Design review of the part built by this model. Coordinates are the model's own, in mm. A direction names the side the tool comes from. Coordinates: 2 decimals unless noted, no trailing zeros. Write each loop counter-clockwise with the first axis right and the second up, starting at its lowest first coordinate (ties: lowest second). Pieces come first, ordered by that corner, then holes.
Q1. Take a section at D-D, the plane z = -8. Write out the cut boundary in (x, y).
Q2. The part is to be moulded in two halves that separate along Y. For faces 1 (the flat face through (-20, 14, -25)), 2 (the flat face through (-0.706, -46.367, 5.514)), 3 (the flat face through (-5, 27.3, -11)), say which applies: released by +Y, released by -Y, zero draft, split by the parting line, or undercut.
Q3. For pin 1 Ø0.6 at (x, z) = (-21, -27.5) entering from -Y; pin 2 Ø21 at (x, y) = (7.5, -3.5) entering from +Z; pin 3 Ø0.9 at (y, z) = (14.5, -25.5) entering from +X, all flat-tipped, find the tip position at first contact; note any pin that passes through.
Q4. Take a section at C-C, the plane x = 2.5. Write out the cut boundary in (y, z).
Q5. Take a section at A-A, the plane x = -15. Write out the cut boundary in (y, z).
Q6. For L1, parallel to Z at x = -9, y = 11.5; L2, parallel to Y at x = 6.5, z = 4; L3, parallel to Z at x = 7.5, y = 14.5, list the stretches that pass through material, from the lowest coordinate up.
Q7. For faces 4 (the flat face through (-21.014, 17.528, -12.159)), 5 (the flat face through (-11, 14, -20.21)), 6 (the flat face through (-21, 12.15, -25)), 7 (the flat face through (7, -20.2, 11)), 8 (the flat face through (-20, -8, -28)), list the 3-axis set-ups (+Z, -Z, +X, -X, +Y, -Y) from which the entire face can be reached by the end or side of a thin tool; tool diameter is ignored.
Q8. Take a section at B-B, the plane y = 16.5. Write out the cut boundary in (x, z).
from build123d import *

# Parameters (mm, degrees)
F1_DEPTH  = 20
F0_W      = 12
F0_H      = 10
F2_DEPTH  = 20
F4_DEPTH  = 2
F8_DEPTH  = 3
F10_DEPTH = 2


with BuildPart() as f1:
    # F0 (on Right) → F1 (new body)
    with BuildSketch(Plane.YZ):
        with BuildLine():
            ThreePointArc((-9.7216395426, -22.7567306352), (3.9984194059, -3.7830302321), (27.3, -6.0803474404))
            Line((27.3, -6.0803474404), (27.3, 1.2904210016))
            Line((27.3, 1.2904210016), (20.2, 1.2904210016))
            Line((20.2, 1.2904210016), (-20.2, 1.2904210016))
            Line((-20.2, 1.2904210016), (-27.3, 1.2904210016))
            Line((-27.3, 1.2904210016), (-33.1852941176, 1.2904210016))
            Line((-33.1852941176, 1.2904210016), (-14.8038696072, -17.5481150452))
            Line((-14.8038696072, -17.5481150452), (-9.7216395426, -22.7567306352))
        make_face()
        with BuildLine():
            Line((-42.245950674, 1.2904210016), (-33.1852941176, 1.2904210016))
            Line((-33.1852941176, 1.2904210016), (-27.3, 1.2904210016))
            Line((-27.3, 1.2904210016), (-27.3, 21.2904210016))
            Line((-27.3, 21.2904210016), (-41.9619835647, 21.2904210016))
            ThreePointArc((-41.9619835647, 21.2904210016), (-43.092993443, 21.0690567559), (-44.0570932222, 20.4376321051))
            Line((-44.0570932222, 20.4376321051), (-50.5527888965, 14.0995525758))
            ThreePointArc((-50.5527888965, 14.0995525758), (-51.4574530171, 11.989182758), (-50.6048903424, 9.8572318148))
            Line((-50.6048903424, 9.8572318148), (-42.245950674, 1.2904210016))
        make_face()
    extrude(amount=F1_DEPTH)

    # F0 (on Right) → F2 (join)
    with BuildSketch(Plane.YZ):
        with BuildLine():
            ThreePointArc((-9.7216395426, -22.7567306352), (3.9984194059, -3.7830302321), (27.3, -6.0803474404))
            Line((27.3, -6.0803474404), (27.3, 1.2904210016))
            Line((27.3, 1.2904210016), (20.2, 1.2904210016))
            Line((20.2, 1.2904210016), (-20.2, 1.2904210016))
            Line((-20.2, 1.2904210016), (-27.3, 1.2904210016))
            Line((-27.3, 1.2904210016), (-33.1852941176, 1.2904210016))
            Line((-33.1852941176, 1.2904210016), (-14.8038696072, -17.5481150452))
            Line((-14.8038696072, -17.5481150452), (-9.7216395426, -22.7567306352))
        make_face()
        with BuildLine():
            ThreePointArc((24.3, -35.2095789984), (26.4213203436, -34.3308993419), (27.3, -32.2095789984))
            Line((27.3, -32.2095789984), (27.3, -6.0803474404))
            ThreePointArc((27.3, -6.0803474404), (3.9984194059, -3.7830302321), (-9.7216395426, -22.7567306352))
            Line((-9.7216395426, -22.7567306352), (2.4290441176, -35.2095789984))
            Line((2.4290441176, -35.2095789984), (24.3, -35.2095789984))
        make_face()
        with Locations((13.65, -25.2095789984)):
            Rectangle(F0_W, F0_H, mode=Mode.SUBTRACT)
        with BuildLine():
            Line((-42.245950674, 1.2904210016), (-33.1852941176, 1.2904210016))
            Line((-33.1852941176, 1.2904210016), (-27.3, 1.2904210016))
            Line((-27.3, 1.2904210016), (-27.3, 21.2904210016))
            Line((-27.3, 21.2904210016), (-41.9619835647, 21.2904210016))
            ThreePointArc((-41.9619835647, 21.2904210016), (-43.092993443, 21.0690567559), (-44.0570932222, 20.4376321051))
            Line((-44.0570932222, 20.4376321051), (-50.5527888965, 14.0995525758))
            ThreePointArc((-50.5527888965, 14.0995525758), (-51.4574530171, 11.989182758), (-50.6048903424, 9.8572318148))
            Line((-50.6048903424, 9.8572318148), (-42.245950674, 1.2904210016))
        make_face()
    extrude(amount=-F2_DEPTH)

    # F3 (on face) → F4 (join)
    with BuildSketch(Plane(origin=(-20, 0, 0), x_dir=(0, -1, 0), z_dir=(-1, 0, 0))):
        with BuildLine():
            Line((-2.4290441176, -35.2095789984), (14.8038696072, -17.5481150452))
            Line((14.8038696072, -17.5481150452), (33.1852941176, 1.2904210016))
            Line((33.1852941176, 1.2904210016), (42.245950674, 1.2904210016))
            Line((42.245950674, 1.2904210016), (50.6048903424, 9.8572318148))
            ThreePointArc((50.6048903424, 9.8572318148), (51.4574530171, 11.989182758), (50.5527888965, 14.0995525758))
            Line((50.5527888965, 14.0995525758), (44.0570932222, 20.4376321051))
            ThreePointArc((44.0570932222, 20.4376321051), (43.092993443, 21.0690567559), (41.9619835647, 21.2904210016))
            Line((41.9619835647, 21.2904210016), (27.3, 21.2904210016))
            Line((27.3, 21.2904210016), (27.3, 1.2904210016))
            Line((27.3, 1.2904210016), (-27.3, 1.2904210016))
            Line((-27.3, 1.2904210016), (-27.3, -32.2095789984))
            ThreePointArc((-27.3, -32.2095789984), (-26.4213203436, -34.3308993419), (-24.3, -35.2095789984))
            Line((-24.3, -35.2095789984), (-2.4290441176, -35.2095789984))
        make_face()
        Polygon((-19.65, -30.2095789984), (-19.65, -20.2095789984), (-15.15, -20.2095789984), (-13.65, -20.2095789984), (-12.15, -20.2095789984), (-7.65, -20.2095789984), (-7.65, -30.2095789984), (-12.15, -30.2095789984), (-15.15, -30.2095789984), align=None, mode=Mode.SUBTRACT)
        with BuildLine():
            ThreePointArc((-2.4290441176, -35.2095789984), (10.8667381723, -30.9446299941), (14.8038696072, -17.5481150452))
            Line((14.8038696072, -17.5481150452), (-2.4290441176, -35.2095789984))
        make_face()
        Polygon((-13.65, -20.2095789984), (-15.15, -20.2095789984), (-15.15, -30.2095789984), (-12.15, -30.2095789984), (-12.15, -20.2095789984), align=None)
    extrude(amount=F4_DEPTH)

    # F7 (on offset) → F8 (join)
    with BuildSketch(Plane.YZ.offset(8)):
        with BuildLine():
            Line((-24.1, 21.2904210016), (-27.3, 21.2904210016))
            Line((-27.3, 21.2904210016), (-27.3, 1.2904210016))
            Line((-27.3, 1.2904210016), (-24.1, 1.2904210016))
            Line((-24.1, 1.2904210016), (-24.1, 4.3404210016))
            ThreePointArc((-24.1, 4.3404210016), (-26.35, 6.5904210016), (-24.1, 8.8404210016))
            Line((-24.1, 8.8404210016), (-24.1, 13.7404210016))
            ThreePointArc((-24.1, 13.7404210016), (-26.35, 15.9904210016), (-24.1, 18.2404210016))
            Line((-24.1, 18.2404210016), (-24.1, 21.2904210016))
        make_face()
        with BuildLine():
            Line((-20.2, 21.2904210016), (-24.1, 21.2904210016))
            Line((-24.1, 21.2904210016), (-24.1, 18.2404210016))
            ThreePointArc((-24.1, 18.2404210016), (-22.5090097423, 17.5814112593), (-21.85, 15.9904210016))
            ThreePointArc((-21.85, 15.9904210016), (-22.5090097423, 14.3994307439), (-24.1, 13.7404210016))
            Line((-24.1, 13.7404210016), (-24.1, 8.8404210016))
            ThreePointArc((-24.1, 8.8404210016), (-22.5090097423, 8.1814112593), (-21.85, 6.5904210016))
            ThreePointArc((-21.85, 6.5904210016), (-22.5090097423, 4.9994307439), (-24.1, 4.3404210016))
            Line((-24.1, 4.3404210016), (-24.1, 1.2904210016))
            Line((-24.1, 1.2904210016), (-20.2, 1.2904210016))
            Line((-20.2, 1.2904210016), (-20.2, 21.2904210016))
        make_face()
        with BuildLine():
            Line((20.2, 21.2904210016), (20.2, 1.2904210016))
            Line((20.2, 1.2904210016), (24.1, 1.2904210016))
            Line((24.1, 1.2904210016), (24.1, 4.3404210016))
            ThreePointArc((24.1, 4.3404210016), (21.85, 6.5904210016), (24.1, 8.8404210016))
            Line((24.1, 8.8404210016), (24.1, 13.7404210016))
            ThreePointArc((24.1, 13.7404210016), (21.85, 15.9904210016), (24.1, 18.2404210016))
            Line((24.1, 18.2404210016), (24.1, 21.2904210016))
            Line((24.1, 21.2904210016), (20.2, 21.2904210016))
        make_face()
        with BuildLine():
            Line((24.1, 4.3404210016), (24.1, 1.2904210016))
            Line((24.1, 1.2904210016), (27.3, 1.2904210016))
            Line((27.3, 1.2904210016), (27.3, 21.2904210016))
            Line((27.3, 21.2904210016), (24.1, 21.2904210016))
            Line((24.1, 21.2904210016), (24.1, 18.2404210016))
            ThreePointArc((24.1, 18.2404210016), (25.6909902577, 17.5814112593), (26.35, 15.9904210016))
            ThreePointArc((26.35, 15.9904210016), (25.6909902577, 14.3994307439), (24.1, 13.7404210016))
            Line((24.1, 13.7404210016), (24.1, 8.8404210016))
            ThreePointArc((24.1, 8.8404210016), (25.6909902577, 8.1814112593), (26.35, 6.5904210016))
            ThreePointArc((26.35, 6.5904210016), (25.6909902577, 4.9994307439), (24.1, 4.3404210016))
        make_face()
    extrude(amount=-F8_DEPTH)

    # F9 (on face) → F10 (cut)
    with BuildSketch(Plane(origin=(-22, 0, 0), x_dir=(0, -1, 0), z_dir=(-1, 0, 0))):
        Polygon((-19.9727848101, -3.8804650743), (-12.15, -20.2095789984), (-9.9, -20.2095789984), (-20.2, 1.2904210016), (-23.75, 1.2904210016), (-17.4, -20.2095789984), (-15.15, -20.2095789984), align=None)
    extrude(amount=-F10_DEPTH, mode=Mode.SUBTRACT)


solid = f1.part
Responses:
1. outline: (-22, -24.12) - (20, -24.12) - (20, -2.35) - (0, -2.35) - (0, 27.3) - (-22, 27.3) - (-22, 21.01) - (-20, 21.01) - (-20, 18.76) - (-22, 18.76) - (-22, 18) - (-20, 18) - (-20, 15.75) - (-22, 15.75) - close
2. face 1: undercut
2. face 2: released by -Y
2. face 3: released by +Y
3. pin 1: stops at y = -13.53
3. pin 2: stops at z = 1.29
3. pin 3: stops at x = -20
4. outline: (-50.6, 9.86) - (-42.25, 1.29) - (-33.19, 1.29) - (-9.72, -22.76) arc R23.5 cw to (27.3, -6.08) - (27.3, 1.29) - (-27.3, 1.29) - (-27.3, 21.29) - (-41.96, 21.29) arc R3 ccw to (-44.06, 20.44) - (-50.55, 14.1) arc R3 ccw to start
5. outline: (-50.6, 9.86) - (-42.25, 1.29) - (-33.19, 1.29) - (2.43, -35.21) - (24.3, -35.21) arc R3 ccw to (27.3, -32.21) - (27.3, 1.29) - (-27.3, 1.29) - (-27.3, 21.29) - (-41.96, 21.29) arc R3 ccw to (-44.06, 20.44) - (-50.55, 14.1) arc R3 ccw to start; hole (7.65, -30.21) - (19.65, -30.21) - (19.65, -20.21) - (7.65, -20.21) - close
6. L1: z = -35.21 to -30.21, -20.21 to 1.29
6. L2: y = -44.89 to -20.2, 20.2 to 27.3
6. L3: z = -1.72 to 1.29
7. face 4: -X
7. face 5: +X
7. face 6: +X, -X
7. face 7: +Z, +X, -X
7. face 8: -Z, +X, -Y
8. outline: (-22, -35.21) - (0, -35.21) - (0, -30.21) - (-22, -30.21) - close; (-22, -15.64) - (-20, -15.64) - (-20, -20.21) - (0, -20.21) - (0, -1.88) - (20, -1.88) - (20, 1.29) - (-22, 1.29) - (-22, -6.43) - (-20, -6.43) - (-20, -11.13) - (-22, -11.13) - close
